CAD build for the part. Positions are in the model's coordinates, mm. A direction names the side the tool comes from. Give positions to 0.01 mm unless a question says otherwise; leave off trailing zeros. Write each loop counter-clockwise with the first axis right and the second up, starting at its lowest first coordinate (ties: lowest second). Pieces come first, ordered by that corner, then holes. Notation, with made-up numbers: (64, 41) - (112, 41) arc R25 cw to (112, 57) - close; hole circle Ø10 at (-19, 87). An arc over 180 degrees is marked (long way). Put each result on its own line as item: value. Start each with the question number.
1. Cut at C-C on y = 52. List the corners of the cut face in (x, z), and give its area (3 significant figures).
2. Wall check: line 1 (Z direction, x = 16.5, y = 44); line 2 (Z direction, x = 48, y = 56). Give the ranges that are in metal, low to high.
3. Cut at B-B on x = 101.5. List the corners of the cut face in (y, z).
4. Tool access for faces 1 (the flat face through (0, 41, 3)), 2 (the flat face through (79, 18.25, 12)), 3 (the flat face through (26.25, 31, 10)): list every direction of +Z, -Z, +X, -X, +Y, -Y with a clear straight run to the whole face (end or side of a thin tool).
5. Cut at D-D on x = 54. List the corners of the cut face in (y, z), and give its area (3 significant figures).
6. Cut at A-A on z = 14.25. List the corners of the cut face in (x, y).
7. Drop flat-ended pins along their axis: pin 1 (4 mm diameter, centred on y = 47, z = 11.5, fed in from +X); pin 2 (6 mm diameter, centred on y = 32, z = 12, fed in from -X); pin 3 (1.5 mm diameter, centred on x = 36.5, y = 21, fed in from +Z). Give the stop position or say it passes through.
Autodesk Inventor part; units mm, degrees
ref_plane "작업 평면1" through (95.75, 0, 0) normal (1, 0, 0) x (0, 0, -1)
ref_plane "작업 평면2" through (26.25, 0, 0) normal (-1, 0, 0) x (0, 0, 1)
ref_plane "YZ Plane" through (0, 0, 0) normal (1, 0, 0) x (0, 1, 0)
sketch "스케치1" plane through (0, 0, 0) normal (0, 0, 1) x (1, 0, 0)
  line L0 (0, 0) -> (122, 0)
  line L1 (122, 0) -> (122, 80)
  line L2 (122, 80) -> (0, 80)
  line L3 (0, 80) -> (0, 0)
  dimension "d0" = 80
  dimension "d1" = 122
extrude "돌출1" add sketch "스케치1" along normal blind 7.8
sketch "스케치2" plane through (0, 0, 7.8) normal (0, 0, 1) x (1, 0, 0)
  line L0 (26.25, 61.75) -> (95.75, 61.75)
  line L1 (95.75, 61.75) -> (95.75, 18.25)
  line L2 (95.75, 18.25) -> (26.25, 18.25)
  line L3 (26.25, 18.25) -> (26.25, 61.75)
  line L4 (0, 80) -> (0, 0)
  line L5 (0, 0) -> (122, 0)
  dimension "d4" = 43.5
  dimension "d5" = 69.5
  dimension "d6" = 26.25
  dimension "d7" = 18.25
ref_plane "작업 평면1" through (95.75, 0, 0) normal (1, 0, 0) x (0, 0, -1)
sketch "스케치3" plane through (95.75, 0, 0) normal (1, 0, 0) x (0, 0, -1)
  line L0 (-7.8, 61.75) -> (-7.8, 18.25)
  line L1 (-7.8, 61.75) -> (-15.6034, 18.25)
  line L2 (-15.6034, 18.25) -> (-7.8, 18.25)
  point P0 (0, 0)
  dimension "d9" = 10.17
extrude "돌출2" add sketch "스케치3" against normal blind 34.7
ref_plane "작업 평면2" through (26.25, 0, 0) normal (-1, 0, 0) x (0, 0, 1)
sketch "스케치4" plane through (26.25, 0, 0) normal (-1, 0, 0) x (0, 0, 1)
  line L0 (7.8, 18.25) -> (7.8, 61.75)
  line L1 (7.8, 18.25) -> (15.6034, 18.25)
  line L2 (15.6034, 18.25) -> (7.8, 61.75)
  point P0 (0, 0)
extrude "돌출3" add sketch "스케치4" against normal blind 34.7
chamfer "모따기1" distance 15 distance2 2 1 edges at (122, 40, 7.8) measured on face at (61.0167, 73.9167, 7.8)
chamfer "모따기2" distance 15 distance2 2 1 edges at (0, 40, 7.8) measured on face at (8.75, 47.25, 7.8)
chamfer "모따기3" distance 13 distance2 2 1 edges at (61, 80, 7.8) measured on face at (61.0167, 73.9167, 7.8)
chamfer "모따기4" distance 13 distance2 2 1 edges at (61, 0, 7.8) measured on face at (60.9833, 6.0833, 7.8)
fillet "모깎기1" radius 10 8 edges at (114.5, 73.5, 6.8) (61, 67, 7.8) (107, 40, 7.8) (114.5, 6.5, 6.8) (61, 13, 7.8) (15, 40, 7.8) (7.5, 6.5, 6.8) (7.5, 73.5, 6.8)
properties part number "스위치2"
Report:
1. outline: (0, 0) - (122, 0) - (122, 5.8) - (107.66, 7.71) arc R10 ccw to (106.34, 7.8) - (95.75, 7.8) - (95.75, 9.55) - (61.05, 9.55) - (61.05, 7.8) - (60.95, 7.8) - (60.95, 9.55) - (26.25, 9.55) - (26.25, 7.8) - (15.66, 7.8) arc R10 ccw to (14.34, 7.71) - (0, 5.8) - close
1. area: 1,040 mm²
2. line 1: z = 0 to 7.8
2. line 2: z = 0 to 8.83
3. outline: (0, 0) - (80, 0) - (80, 5.8) - (67.76, 7.68) arc R10 ccw to (66.24, 7.8) - (13.76, 7.8) arc R10 ccw to (12.24, 7.68) - (0, 5.8) - close
4. face 1: +Z, -Z, -X, +Y, -Y
4. face 2: +Z, +X, -X, -Y
4. face 3: +Z, -X, +Y, -Y
5. outline: (0, 0) - (80, 0) - (80, 5.8) - (67.76, 7.68) arc R10 ccw to (66.24, 7.8) - (61.75, 7.8) - (18.25, 15.6) - (18.25, 7.8) - (13.76, 7.8) arc R10 ccw to (12.24, 7.68) - (0, 5.8) - close
5. area: 768 mm²
6. outline: (26.25, 18.25) - (60.95, 18.25) - (60.95, 25.79) - (26.25, 25.79) - close; (61.05, 18.25) - (95.75, 18.25) - (95.75, 25.79) - (61.05, 25.79) - close
7. pin 1: stops at x = 95.75
7. pin 2: stops at x = 26.25
7. pin 3: stops at z = 15.24
